from build123d import *

# Parameters (mm, degrees)
F0_W      = 819.15
F0_H      = 101.6
F1_DEPTH  = 25.4
F2_R      = 4.5640625
F3_DEPTH  = 50.8
F4_R      = 12.7
F5_DEPTH  = 19.05
F7_DEPTH  = 25.4
F9_D      = 6.35
F9_DEPTH  = 12.7
F9_TIP    = 1.9077324654
F10_W     = 12.7
F10_H     = 12.7
F11_DEPTH = 50.8
F12_W     = 615.95
F12_H     = 25.4
F13_DEPTH = 25.4


# Not quite as in the source:
# - a feature names something its author has since deleted; it is built from what else it names


with BuildPart() as f1:
    # F0 (on Front) → F1 (new body)
    with BuildSketch(Plane.XZ):
        with Locations((409.575, 50.8)):
            Rectangle(F0_W, F0_H)
    extrude(amount=F1_DEPTH)

    # F2 (on face) → F3 (cut)
    with BuildSketch(Plane(origin=(0, 0, 0), x_dir=(0, -1, 0), z_dir=(-1, 0, 0))):
        with Locations((12.7, 76.2)):
            Circle(F2_R)
    extrude(amount=-F3_DEPTH, mode=Mode.SUBTRACT)

    # F4 (on Front) → F5 (cut)
    with BuildSketch(Plane.XZ):
        with Locations((765.175, 76.2)):
            Circle(F4_R)
        with Locations((53.975, 76.2)):
            Circle(F4_R)
    extrude(amount=F5_DEPTH, mode=Mode.SUBTRACT)

    # F6 (on face) → F7 (cut, through all)
    with BuildSketch(Plane(origin=(0, 0, 0), x_dir=(-1, 0, 0), z_dir=(0, 1, 0))):
        Polygon((-676.275, 19.05), (-676.275, 0), (-142.875, 0), (-142.875, 19.05), (-244.475, 19.05), (-244.475, 38.1), (-574.675, 38.1), (-574.675, 19.05), align=None)
    extrude(amount=-F7_DEPTH, mode=Mode.SUBTRACT)

    # F9
    with Locations(Plane.XY.offset(101.6)):
        with Locations((20.6375, -12.7), (798.5125, -12.7)):
            Hole(F9_D / 2, depth=F9_DEPTH)
            with Locations((0, 0, -(F9_DEPTH + F9_TIP / 2))):  # 118° drill point
                Cone(0, F9_D / 2, F9_TIP, mode=Mode.SUBTRACT)

    # F10 (on Top) → F11 (join)
    with BuildSketch(Plane.XY):
        with Locations((-6.35, -12.7)):
            Rectangle(F10_W, F10_H)
        with Locations((825.5, -12.7)):
            Rectangle(F10_W, F10_H)
    extrude(amount=F11_DEPTH)

    # F12 (on face) → F13 (join)
    with BuildSketch(Plane(origin=(0, 0, 0), x_dir=(-1, 0, 0), z_dir=(0, 1, 0))):
        with Locations((-409.575, 73.025)):
            Rectangle(F12_W, F12_H)
    extrude(amount=F13_DEPTH)


solid = f1.part
Input: part model. Units: mm. Frame: model coordinates. A direction names the side the tool comes from. Coordinates: 2 decimals unless noted, no trailing zeros. Loops run counter-clockwise (first coordinate to the right, second up) from the corner with the lowest first, then second, coordinate; pieces in that order, holes last. Notation, with made-up numbers: (6.25, 69.25) -> (59.25, 69.25) arc R14 cw to (59.25, 76.25) -> close; hole circle Ø10 at (42.5, -7). An arc over 180 degrees is marked (long way). Write item = value, one per line. Start each with the question number.
Item 1: First-contact query: P1, Ø2, axis at y = 10, z = 69.5, coming from the +X side; P2, Ø12.5, axis at y = 6.5, z = 72.5, coming from the -X side; P3, Ø12, axis at y = 3, z = 11, coming from the -X side; P4, Ø8.5, axis at x = 798.51, y = -12.7, coming from the +Z side. Flat tips, straight axial feed; report the tip coordinate or a pass-through.
Item 2: Mould query, pull axis X, two halves, no side actions, for faces 1 (the face through (762.422, -9.392, 63.802)), 2 (the face through (404, -13, 101.6)), 3 (the face through (765, -19.05, 76)), 4 (the face through (717.55, 13, 73)). Classes: pulls with the +X half, pulls with the -X half, needs draft (parallel to the pull), parting line crosses it, or undercut.
Item 3: Cut plane C-C, the plane x = 520. Return loops of the section in (y, z) (3 decimals).
Item 4: Cut plane A-A, the plane z = 27. Return loops of the section in (x, y) (3 decimals).
Item 5: Reachability of faces 5 (the face through (676.275, -13, 10)), 6 (the face through (101.6, 13, 73)), 7 (the face through (65.71, -9.39, 71.34)), 8 (the face through (414, 13, 60.325)), 9 (the face through (404, -25.4, 63)) from +Z, -Z, +X, -X, +Y, -Y: full face, straight path, thin tool, end or side. Return the list, or none.
Item 6: Cut plane D-D, the plane y = 10. Return loops of the section in (x, z) (3 decimals), plus the area to 3 significant figures.
Item 7: Cut plane B-B, the plane x = 631.5. Return loops of the section in (y, z) (3 decimals).
Item 8: Material intervals for line 1 (Z direction, x = 28, y = -12); line 2 (X direction, y = -5, z = 7.5) (3 decimals); line 3 (X direction, y = -10, z = 76), sorted ascending.
Ans:
q1.P1 = 717.55
q1.P2 = 101.6
q1.P3 = 0
q1.P4 = 101.6
q2.face_1 = undercut
q2.face_2 = needs draft
q2.face_3 = undercut
q2.face_4 = pulls with the +X half
q3.outline = (-25.4, 38.1) -> (0, 38.1) -> (0, 60.325) -> (25.4, 60.325) -> (25.4, 85.725) -> (0, 85.725) -> (0, 101.6) -> (-25.4, 101.6) -> close
q4.outline = (-12.7, -19.05) -> (0, -19.05) -> (0, -25.4) -> (244.475, -25.4) -> (244.475, 0) -> (0, 0) -> (0, -6.35) -> (-12.7, -6.35) -> close; (574.675, -25.4) -> (819.15, -25.4) -> (819.15, -19.05) -> (831.85, -19.05) -> (831.85, -6.35) -> (819.15, -6.35) -> (819.15, 0) -> (574.675, 0) -> close
q5.face_5 = -Z, +Y, -Y
q5.face_6 = +Z, -Z, -X, +Y
q5.face_7 = +Y
q5.face_8 = -Z, +X, -X, +Y
q5.face_9 = +Z, -Z, +X, -X, -Y
q6.outline = (101.6, 60.325) -> (717.55, 60.325) -> (717.55, 85.725) -> (101.6, 85.725) -> close
q6.area = 15,600 mm²
q7.outline = (-25.4, 19.05) -> (0, 19.05) -> (0, 60.325) -> (25.4, 60.325) -> (25.4, 85.725) -> (0, 85.725) -> (0, 101.6) -> (-25.4, 101.6) -> close
q8.line_1 = 0 to 71.69, 80.71 to 101.6
q8.line_2 = 0 to 142.875, 676.275 to 819.15
q8.line_3 = 66.67 to 752.48, 777.87 to 819.15
